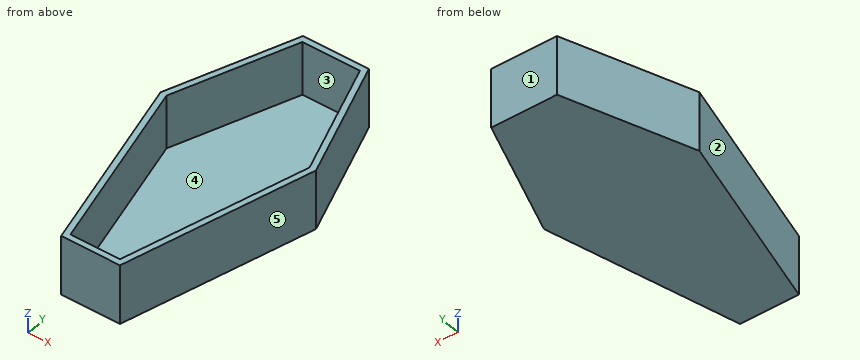
```python
from build123d import *

# Parameters (mm, degrees)
F1_DEPTH = 25.4
F2_T     = -2.54


# Not quite as in the source:
# - a feature of the source that left no trace in its solid (it failed there, or was rolled back) is left out


with BuildPart() as f1:
    # F0 (on Top) → F1 (new body)
    with BuildSketch(Plane.XY):
        Polygon((0, 74.6065601707), (0, -57.7306561172), (12.4910129234, -57.7306561172), (33.0843068659, 21.9417531043), (13.9860804434, 74.6065601707), align=None)
        Polygon((-12.4910129234, -57.7306561172), (0, -57.7306561172), (0, 74.6065601707), (-13.9860804434, 74.6065601707), (-33.0843068659, 21.9417531043), align=None)
    extrude(amount=F1_DEPTH)

    # F2
    f2_openings = [f1.faces().sort_by_distance(p)[0] for p in [
        (0, 11.07211, 25.4),
    ]]
    offset(amount=F2_T, openings=f2_openings)


solid = f1.part
```
Geometry: final body of the model. Coordinates: model frame, mm. Face numbers are marked on the shaded views. A direction names the side the tool comes from. Round coordinates to 2 decimals unless told otherwise and drop trailing zeros. Write each loop counter-clockwise with the first axis right and the second up, starting at its lowest first coordinate (ties: lowest second). Pieces come first, ordered by that corner, then holes.
Item 1: Material intervals for L1, parallel to Y at x = -1, z = 17.5; L2, parallel to Z at x = -19.5, y = 20.5; L3, parallel to X at y = -13, z = 15.5, sorted ascending.
Item 2: Pin query (flat end, axial travel): P1, Ø8, axis at y = 31.5, z = 8.5, coming from the +X side; P2, Ø8, axis at y = 32.5, z = 16.5, coming from the +X side; P3, Ø10, axis at x = 9, y = -22.5, coming from the +Z side; P4, Ø4, axis at x = 9, y = 61, coming from the -Z side. Return the tip coordinate at first contact, or that it passes through.
Item 3: Set-up query: the marked faces 4 and 5. Return all of +Z, -Z, +X, -X, +Y, -Y with unobstructed straight access to the full face (end or side cutting, diameter ignored); none if empty.
Item 4: Section query C-C (x = 15.5). Return loops of the section in (y, z), plus the area to 3 significant figures.
Item 5: Mould query, pull axis Y, two halves, no side actions, for the marked faces 1, 2 and 3. Classes: +Y half, -Y half, draft (parallel to the pull), parting line (faces both ways), or undercut.
Item 6: Section query B-B (y = 11). Return loops of the section in (x, z), plus the area to 3 significant figures.
Item 7: Section query A-A (z = 7.25). Return loops of the section in (x, y), plus the area to 3 significant figures.
Completed:
1. L1: y = -57.73 to -55.19, 72.07 to 74.61
1. L2: z = 0 to 2.54
1. L3: x = -24.05 to -21.43, 21.43 to 24.05
2. P1: stops at x = 31.07
2. P2: stops at x = 30.71
2. P3: stops at z = 2.54
2. P4: stops at z = 0
3. face 4: +Z
3. face 5: +Z, -Z, +X, -Y
4. outline: (-46.09, 0) - (70.43, 0) - (70.43, 25.4) - (62.98, 25.4) - (62.98, 2.54) - (-35.94, 2.54) - (-35.94, 25.4) - (-46.09, 25.4) - close
4. area: 698 mm2
5. face 1: +Y half
5. face 2: -Y half
5. face 3: undercut
6. outline: (-30.26, 0) - (30.26, 0) - (30.26, 25.4) - (27.63, 25.4) - (27.63, 2.54) - (-27.63, 2.54) - (-27.63, 25.4) - (-30.26, 25.4) - close
6. area: 274 mm2
7. outline: (-33.08, 21.94) - (-12.49, -57.73) - (12.49, -57.73) - (33.08, 21.94) - (13.99, 74.61) - (-13.99, 74.61) - close; hole (-30.43, 21.82) - (-10.52, -55.19) - (10.52, -55.19) - (30.43, 21.82) - (12.21, 72.07) - (-12.21, 72.07) - close
7. area: 814 mm2
